Verification items for the finished model (mm, model axes). A direction names the side the tool comes from. Round coordinates to 2 decimals unless told otherwise and drop trailing zeros. Write each loop counter-clockwise with the first axis right and the second up, starting at its lowest first coordinate (ties: lowest second). Pieces come first, ordered by that corner, then holes. Notation, with made-up numbers: M 72,78 L 121,78 A15 cw 121,87 Z; hole C 32.5,-18.75 d6. An arc over 180 degrees is marked long. Answer in a Markdown table with one row per item. Add a question column.
1. Sectioned sample at A-A on y = 159. Record the cut outline in (x, z), plus the area to 3 significant figures.
2. Material ranges on probe 1 along X at (y, z) = (96, 0); probe 2 along X at (y, z) = (179, 125.5); probe 3 along X at (y, z) = (84, -103), recorded low to high.
3. Go/stop test with flat-tipped pins: pin 1 Ø5 at (y, z) = (60.5, -69.5) entering from +X; pin 2 Ø1 at (x, z) = (14.5, -4.5) entering from +Y; pin 3 Ø10 at (x, z) = (-247.5, 98) entering from -Y. Record where each tip stops, or that it passes through.
4. Sectioned sample at C-C on x = 0. Record the cut outline in (y, z).
5. Sectioned sample at B-B on x = 355. Record the cut outline in (y, z).
6. Draft check along Z on faces 6 (the flat face through (2, -5, -150)), 7 (the flat face through (217.5, 105, 2)), 8 (the flat face through (-1, 0, 1)). Enter one of: pulls with the +Z half, pulls with the -Z half, needs draft (parallel to the pull), parting line crosses it, or undercut.
7. Sectioned sample at D-D on z = 0. Count the separate pieces of the cut face and the enclosed holes in it, plus the area to 3 significant figures.
8. Set-up check for faces 1 (the cylindrical face through (-181.486, 5.703, 2.1)), 2 (the flat face through (-328, 208, 2)), 3 (the flat face through (-475, 223, 2)), 4 (the cylindrical face through (-4.95, 83.81, 112.39)), 5 (the flat face through (384, 208, 2)): record each of +Z, -Z, +X, -X, +Y, -Y from which the full face is reachable in a straight line by a thin tool's end or side.
```python
from build123d import *

# Parameters (mm, degrees)
BOSS_EXTRUDE1_DEPTH = 150
FILLET1_R           = 20
FILLET2_R           = 50
SKETCH2_R           = 25
CUT_EXTRUDE1_DEPTH  = 566.640345096
SKETCH3_R           = 112.5
SKETCH3_R_2         = 58.5
BOSS_EXTRUDE2_DEPTH = 170


with BuildPart() as part:
    # Sketch1 → Boss-Extrude1 (new, symmetric)
    with BuildSketch(Plane.XY):
        Polygon((-187.5, 0), (187.5, 0), (187.5, 238), (475, 238), (475, 208), (217.5, 208), (217.5, -30), (-217.5, -30), (-217.5, 208), (-475, 208), (-475, 238), (-187.5, 238), align=None)
    extrude(amount=BOSS_EXTRUDE1_DEPTH, both=True)

    # Fillet1
    fillet1_edges = [part.edges().sort_by_distance(p)[0] for p in [
        (-187.5, 0, 0),
        (187.5, 0, 0),
        (217.5, 208, 0),
        (-217.5, 208, 0),
    ]]
    fillet(fillet1_edges, radius=FILLET1_R)

    # Fillet2
    fillet2_edges = [part.edges().sort_by_distance(p)[0] for p in [
        (187.5, 238, 0),
        (217.5, -30, 0),
        (-217.5, -30, 0),
        (-187.5, 238, 0),
    ]]
    fillet(fillet2_edges, radius=FILLET2_R)

    # Sketch2 → Cut-Extrude1 (cut, through all)
    with BuildSketch(Plane(origin=(0, 238, 0), x_dir=(1, 0, 0), z_dir=(0, 1, 0))):
        with Locations(Location((-355, 0, 0), (0, 0, 180))):
            Circle(SKETCH2_R)
        with Locations(Location((355, 0, 0), (0, 0, 270))):
            Circle(SKETCH2_R)
    extrude(amount=-CUT_EXTRUDE1_DEPTH, mode=Mode.SUBTRACT)

    # Sketch3 → Boss-Extrude2 (add)
    with BuildSketch(Plane(origin=(0, 0, 0), x_dir=(1, 0, 0), z_dir=(0, 1, 0))):
        with Locations(Location((0, 0, 0), (0, 0, 90))):
            Circle(SKETCH3_R)
        with Locations(Location((0, 0, 0), (0, 0, 270))):
            Circle(SKETCH3_R_2, mode=Mode.SUBTRACT)
    extrude(amount=BOSS_EXTRUDE2_DEPTH)


solid = part.part
```
Geometry check:
| question | item | result |
|---|---|---|
| 1 | outline | M -217.5,-150 L -187.5,-150 L -187.5,150 L -217.5,150 Z; C 0,0 d225; M 187.5,-150 L 217.5,-150 L 217.5,150 L 187.5,150 Z; hole C 0,0 d117 |
| 1 | area | 47,000 mm2 |
| 2 | probe 1 | x = -217.5 to -187.5, -112.5 to -58.5, 58.5 to 112.5, 187.5 to 217.5 |
| 2 | probe 2 | x = -217.5 to -187.5, 187.5 to 217.5 |
| 2 | probe 3 | x = -217.5 to -187.5, -45.25 to 45.25, 187.5 to 217.5 |
| 3 | pin 1 | stops at x = 217.5 |
| 3 | pin 2 | stops at y = 0 |
| 3 | pin 3 | stops at y = 208 |
| 4 | outline | M -30,-150 L 0,-150 L 0,-112.5 L 170,-112.5 L 170,-58.5 L 0,-58.5 L 0,58.5 L 170,58.5 L 170,112.5 L 0,112.5 L 0,150 L -30,150 Z |
| 5 | outline | M 208,-150 L 238,-150 L 238,-25 L 208,-25 Z; M 208,25 L 238,25 L 238,150 L 208,150 Z |
| 6 | face 6 | pulls with the -Z half |
| 6 | face 7 | needs draft |
| 6 | face 8 | undercut |
| 7 | separate pieces | 3 |
| 7 | enclosed holes | 0 |
| 7 | area | 56,300 mm2 |
| 8 | face 1 | +Z, -Z, +Y |
| 8 | face 2 | +Z, -Z, -X, -Y |
| 8 | face 3 | +Z, -Z, -X, +Y, -Y |
| 8 | face 4 | +Y |
| 8 | face 5 | +Z, -Z, +X, -Y |
